Geometry: see drawing. Coordinates: mm, zero at the bounding-box minimum. Give positions to 0.01 mm unless a question says otherwise; leave off trailing zeros. Loops run counter-clockwise (first coordinate to the right, second up) from the corner with the lowest first, then second, coordinate; pieces in that order, holes last. Notation, with made-up numbers: (-11, 35) - (48, 35) arc R26 cw to (48, 62) - close; hole circle Ø7 at (-15.75, 43.25). An arc over 180 degrees is marked (long way). Use one line per item in the form item = value.
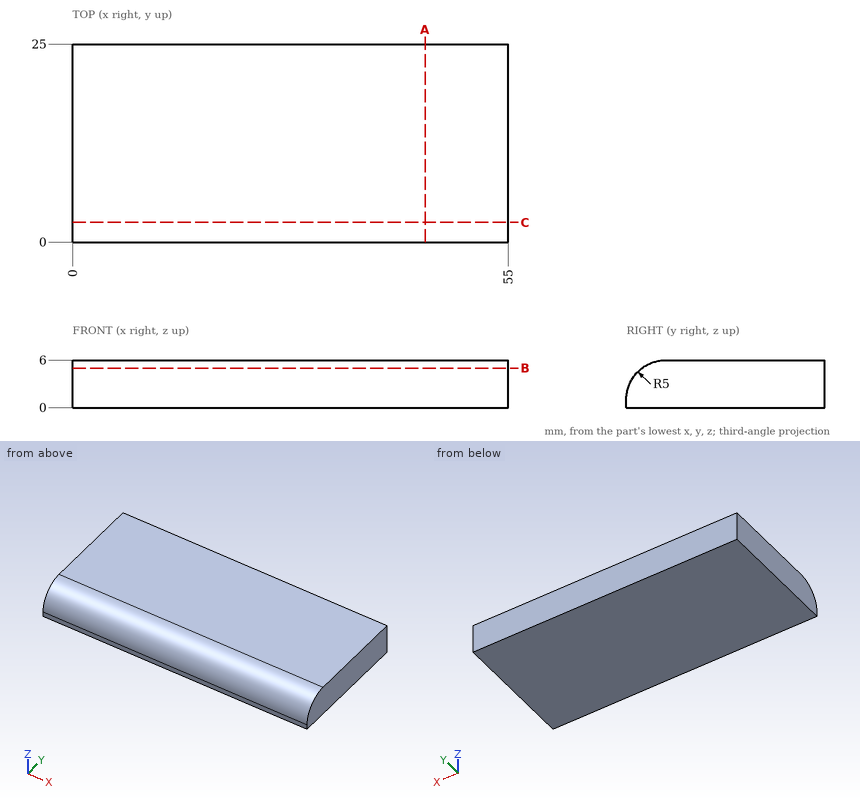
(1) Material intervals for L1, parallel to Y at x = 35.5, z = 1.25; L2, parallel to Y at x = 3.5, z = 4.75, sorted ascending. Write a range as from..to.
Solution:
L1 = 0.01..25
L2 = 1.69..25
(2) Pin query (flat end, axial travel): P1, Ø3, axis at x = 46, z = 3, coming from the -Y side. Return the tip coordinate at first contact, or that it passes through.
Solution:
P1 = 0.03
(3) Cut plane B-B (z = 5). Return the cut outline in (x, y).
Solution:
outline = (0, 2) - (55, 2) - (55, 25) - (0, 25) - close
(4) Cut plane A-A (x = 44.5). Return the cut outline in (y, z), plus the area to 3 significant figures.
Solution:
outline = (0, 0) - (25, 0) - (25, 6) - (5, 6) arc R5 ccw to (0, 1) - close
area = 145 mm2
(5) Cut plane C-C (y = 2.5). Return the cut outline in (x, z).
Solution:
outline = (0, 0) - (55, 0) - (55, 5.33) - (0, 5.33) - close
